from build123d import *

# Parameters (mm, degrees)
BOSS_EXTRUDE1_DEPTH = 0.8128
SKETCH2_R           = 2.413
CUT_EXTRUDE1_DEPTH  = 2.54


with BuildPart() as part:
    # Sketch1 → Boss-Extrude1 (new body)
    with BuildSketch(Plane(origin=(0, 0, 0), x_dir=(-1, 0, 0), z_dir=(0, 0, -1))):
        Polygon((8.385680008, -18.845494556), (5.210680008, -15.670494556), (-3.044319992, -15.670494556), (-3.044319992, -7.415494556), (-6.219319992, -4.240494556), (-12.569319992, -4.240494556), (-15.744319992, -7.415494556), (-15.744319992, -15.670494556), (-23.999319992, -15.670494556), (-27.174319992, -18.845494556), (-27.174319992, -25.195494556), (-23.999319992, -28.370494556), (-15.744319992, -28.370494556), (-15.744319992, -36.625494556), (-12.569319992, -39.800494556), (-6.219319992, -39.800494556), (-3.044319992, -36.625494556), (-3.044319992, -28.370494556), (5.210680008, -28.370494556), (8.385680008, -25.195494556), align=None)
        with BuildLine():
            Line((5.109080019, -24.331894556), (1.502279997, -24.331894556))
            ThreePointArc((1.502279997, -24.331894556), (1.14306976, -24.183104805), (0.994280008, -23.823894568))
            Line((0.994280008, -23.823894568), (0.994280008, -20.217094545))
            ThreePointArc((0.994280008, -20.217094545), (1.14306976, -19.857884308), (1.502279997, -19.709094556))
            Line((1.502279997, -19.709094556), (5.109080019, -19.709094556))
            ThreePointArc((5.109080019, -19.709094556), (5.468290256, -19.857884308), (5.617080008, -20.217094545))
            Line((5.617080008, -20.217094545), (5.617080008, -23.823894568))
            ThreePointArc((5.617080008, -23.823894568), (5.468290256, -24.183104805), (5.109080019, -24.331894556))
        make_face(mode=Mode.SUBTRACT)
        with BuildLine():
            Line((-7.590919981, -24.331894556), (-11.197720003, -24.331894556))
            ThreePointArc((-11.197720003, -24.331894556), (-11.55693024, -24.183104805), (-11.705719992, -23.823894568))
            Line((-11.705719992, -23.823894568), (-11.705719992, -20.217094545))
            ThreePointArc((-11.705719992, -20.217094545), (-11.55693024, -19.857884308), (-11.197720003, -19.709094556))
            Line((-11.197720003, -19.709094556), (-7.590919981, -19.709094556))
            ThreePointArc((-7.590919981, -19.709094556), (-7.231709744, -19.857884308), (-7.082919992, -20.217094545))
            Line((-7.082919992, -20.217094545), (-7.082919992, -23.823894568))
            ThreePointArc((-7.082919992, -23.823894568), (-7.231709744, -24.183104805), (-7.590919981, -24.331894556))
        make_face(mode=Mode.SUBTRACT)
        with BuildLine():
            Line((-11.197720003, -7.009094556), (-7.590919981, -7.009094556))
            ThreePointArc((-7.590919981, -7.009094556), (-7.231709744, -7.157884308), (-7.082919992, -7.517094545))
            Line((-7.082919992, -7.517094545), (-7.082919992, -11.123894568))
            ThreePointArc((-7.082919992, -11.123894568), (-7.231709744, -11.483104805), (-7.590919981, -11.631894556))
            Line((-7.590919981, -11.631894556), (-11.197720003, -11.631894556))
            ThreePointArc((-11.197720003, -11.631894556), (-11.55693024, -11.483104805), (-11.705719992, -11.123894568))
            Line((-11.705719992, -11.123894568), (-11.705719992, -7.517094545))
            ThreePointArc((-11.705719992, -7.517094545), (-11.55693024, -7.157884308), (-11.197720003, -7.009094556))
        make_face(mode=Mode.SUBTRACT)
        with BuildLine():
            Line((-20.290919981, -24.331894556), (-23.897720003, -24.331894556))
            ThreePointArc((-23.897720003, -24.331894556), (-24.25693024, -24.183104805), (-24.405719992, -23.823894568))
            Line((-24.405719992, -23.823894568), (-24.405719992, -20.217094545))
            ThreePointArc((-24.405719992, -20.217094545), (-24.25693024, -19.857884308), (-23.897720003, -19.709094556))
            Line((-23.897720003, -19.709094556), (-20.290919981, -19.709094556))
            ThreePointArc((-20.290919981, -19.709094556), (-19.931709744, -19.857884308), (-19.782919992, -20.217094545))
            Line((-19.782919992, -20.217094545), (-19.782919992, -23.823894568))
            ThreePointArc((-19.782919992, -23.823894568), (-19.931709744, -24.183104805), (-20.290919981, -24.331894556))
        make_face(mode=Mode.SUBTRACT)
        with BuildLine():
            Line((-11.705719992, -36.523894568), (-11.705719992, -32.917094545))
            ThreePointArc((-11.705719992, -32.917094545), (-11.55693024, -32.557884308), (-11.197720003, -32.409094556))
            Line((-11.197720003, -32.409094556), (-7.590919981, -32.409094556))
            ThreePointArc((-7.590919981, -32.409094556), (-7.231709744, -32.557884308), (-7.082919992, -32.917094545))
            Line((-7.082919992, -32.917094545), (-7.082919992, -36.523894568))
            ThreePointArc((-7.082919992, -36.523894568), (-7.231709744, -36.883104805), (-7.590919981, -37.031894556))
            Line((-7.590919981, -37.031894556), (-11.197720003, -37.031894556))
            ThreePointArc((-11.197720003, -37.031894556), (-11.55693024, -36.883104805), (-11.705719992, -36.523894568))
        make_face(mode=Mode.SUBTRACT)
    extrude(amount=-BOSS_EXTRUDE1_DEPTH)

    # Sketch2 → Cut-Extrude1 (cut)
    with BuildSketch(Plane.XY.offset(0.8128)):
        with Locations((-3.305680008, -22.020494556)):
            Circle(SKETCH2_R)
        with Locations((9.394319992, -22.020494556)):
            Circle(SKETCH2_R)
        with Locations((9.394319992, -9.320494556)):
            Circle(SKETCH2_R)
        with Locations((22.094319992, -22.020494556)):
            Circle(SKETCH2_R)
        with Locations((9.394319992, -34.720494556)):
            Circle(SKETCH2_R)
    extrude(amount=-CUT_EXTRUDE1_DEPTH, mode=Mode.SUBTRACT)


solid = part.part
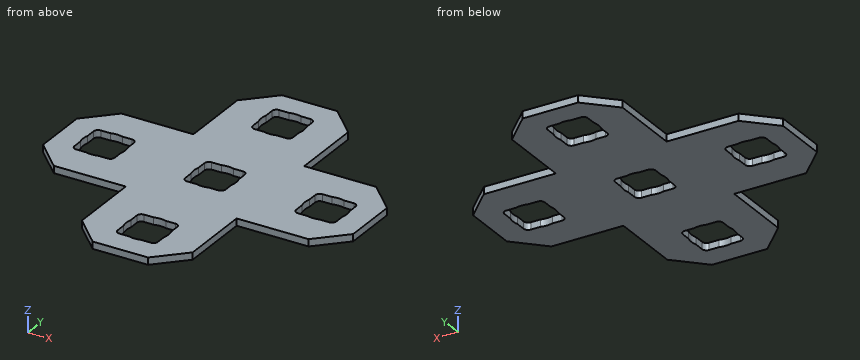
The listing builds one solid part. Answer for the finished solid, in the listing's coordinates (mm). Round coordinates to 2 decimals unless told otherwise and drop trailing zeros. Write each loop counter-clockwise with the first axis right and the second up, starting at its lowest first coordinate (ties: lowest second). Pieces come first, ordered by that corner, then holes. Notation, with made-up numbers: M 26,-12.75 L 74,-12.75 A8 ccw 74,0.25 Z; hole C 37,6.25 d3. An arc over 180 degrees is marked long. Write each question's results on one line, items separated by ' | '. Start each with the question number.
(1) The part is cut by section B-B, the plane x = 22. Write down the section's boundary in (y, z).
(2) The part is cut by section D-D, the plane z = 0.45. Give the number of separate pieces and of enclosed holes in the cut face, and give its area (3 significant figures).
(3) The part is cut by section A-A, the plane y = -36. Write down the section's boundary in (x, z), and give its area (3 significant figures).
(4) Find the intervals of material crossed by line 1 (Y direction, x = 8.5, z = 0.6); line 2 (Y direction, x = 24, z = 0.55); line 3 (Y direction, x = 22, z = 0.55), in increasing order.
(5) The part is cut by section C-C, the plane y = -22. Write down the section's boundary in (x, z), and give its area (3 significant figures).
Worked answers:
1) outline: M -28.37,0 L -24.43,0 L -24.43,0.81 L -28.37,0.81 Z; M -19.61,0 L -15.67,0 L -15.67,0.81 L -19.61,0.81 Z
2) separate pieces: 1 | enclosed holes: 5 | area: 594 mm²
3) outline: M 3.04,0 L 7.08,0 L 7.08,0.81 L 3.04,0.81 Z; M 11.71,0 L 15.74,0 L 15.74,0.81 L 11.71,0.81 Z | area: 6.57 mm²
4) line 1: y = -39.8 to -37.03, -32.41 to -24.33, -19.71 to -11.63, -7.01 to -4.24 | line 2: y = -28.37 to -24.32, -19.72 to -15.67 | line 3: y = -28.37 to -24.43, -19.61 to -15.67
5) outline: M -8.39,0 L -5.72,0 L -5.72,0.81 L -8.39,0.81 Z; M -0.89,0 L 6.98,0 L 6.98,0.81 L -0.89,0.81 Z; M 11.81,0 L 19.68,0 L 19.68,0.81 L 11.81,0.81 Z; M 24.51,0 L 27.17,0 L 27.17,0.81 L 24.51,0.81 Z | area: 17.1 mm²
